Here's how the part is built. I have some questions about the finished solid (model axes, mm). A direction names the side the tool comes from. Coordinates: 2 decimals unless noted, no trailing zeros. Order: outer loops, then holes, each group sorted by start corner. A loop starts at its lowest first (then second) coordinate and runs counter-clockwise, first axis right, second up. Notation, with made-up numbers: (-17.75, 8) - (28.25, 8) arc R9 ccw to (28.25, 12) - close; hole circle Ø1 at (48, 76.5). An arc over 180 degrees is marked (long way). Answer as CSV lines item,"result". Start each with the question number.
Q1. Suppose I cut it at B-B (x = 3.5). Please give me the cut outline in (y, z).
Q2. For faces 1 (the face through (-4, 4, 35)), 2 (the face through (-5, 0, 44.85)), 3 (the face through (3, 0, 59.85)), which set-ups out of +Z, -Z, +X, -X, +Y, -Y let a thin tool reach every point of the face, with its end or its side?
Q3. Suppose I cut it at A-A (y = -3.75). Please give me the cut outline in (x, z), then the cut area to 3 significant figures.
Q4. Suppose I cut it at C-C (z = 20). Please give me the cut outline in (x, y).
Q5. Suppose I cut it at D-D (z = 54.5). Please give me the cut outline in (x, y).
Q6. Thinking about a two-plate mould opening in Y: for faces 4 (the face through (-1.08, 4.88, 17.26)), 5 (the face through (2.44, 0.54, 55.79)), 6 (the face through (-4, 0, 52)), 7 (the face through (-0.424, 0.094, 50.609)), which applies, released by +Y, released by -Y, zero draft, split by the parting line, or undercut?
Q7. I need wall thicknesses on line 1 (X direction, y = 0, z = 56.25); line 2 (Y direction, x = 0, z = 54.25); line 3 (Z direction, x = -4.75, y = 3.25). Which ranges of each line are inside material? Lowest first, please.
Q8. For pin 1 Ø3.5 at (x, y) = (1, 1.5) entering from -Z; pin 2 Ø7 at (y, z) = (0.5, 51) entering from -X; pin 3 Ø4 at (y, z) = (-4, 27) entering from -X, each with a flat end and sliding along its axis, tell me the tip position at first contact or that it passes through.
Autodesk Inventor part; units mm, degrees
ref_plane "作業平面1" through (0, 6, 59.85) normal (0, 1, 0) x (-1, 0, 0)
ref_plane "YZ Plane" through (0, 0, 0) normal (1, 0, 0) x (0, 1, 0)
ref_plane "XZ Plane" through (0, 0, 0) normal (0, 1, 0) x (-1, 0, 0)
sketch "スケッチ1" plane through (0, 0, 0) normal (0, 0, 1) x (1, 0, 0)
  point P0 (0, 0)
sketch "スケッチ2" plane through (0, 0, 0) normal (0, 0, 1) x (1, 0, 0)
  circle A0 centre (0, 0) radius 5
  dimension "d0" = 10
extrude "押し出し1" add sketch "スケッチ2" along normal blind 35
thread "ねじ1"
sketch "スケッチ3" plane through (0, 0, 35) normal (0, 0, 1) x (1, 0, 0)
  point P0 (0, 0)
sketch "スケッチ4" plane through (0, 0, 35) normal (0, 0, 1) x (1, 0, 0)
  circle A0 centre (0, 0) radius 6
  dimension "d5" = 12
extrude "押し出し2" add sketch "スケッチ4" along normal blind 24.85
sketch "スケッチ5" plane through (0, 0, 59.85) normal (0, 0, 1) x (1, 0, 0)
  line L0 (0, 0) -> (0, 6)
  circle A0 centre (0, 0) radius 6
ref_plane "作業平面1" through (0, 6, 59.85) normal (0, 1, 0) x (-1, 0, 0)
sketch "スケッチ9" plane through (0, 0, 59.85) normal (0, 0, 1) x (1, 0, 0)
  point P0 (0, 0)
  point P1 (0, 0)
hole "穴2" at (0, 0, 59.85) direction (0, 0, -1) diameter 5 depth 8 tip angle 118
thread "ねじ3"
sketch "スケッチ10" plane through (0, 0, 59.85) normal (0, 0, 1) x (1, 0, 0)
  arc A0 (-4, 4.4721) -> (-4, -4.4721) centre (0, 0) ccw
  line L0 (-4, 0) -> (-4, 4.4721)
  line L1 (-4, 0) -> (-4, -4.4721)
  dimension "d34" = 12
  dimension "d35" = 4
extrude "押し出し4" cut sketch "スケッチ10" against normal blind 15
properties part number "回転アーム付き計測輪シャフト"
Here are the results:
1,outline,"(-4.87, 35) - (-3.57, 35) - (-3.57, 0) - (3.57, 0) - (3.57, 35) - (4.87, 35) - (4.87, 59.85) - (-4.87, 59.85) - close"
2,face 1,"-Z"
2,face 2,"+Z, -X, +Y, -Y"
2,face 3,"+Z, +X, -X, +Y, -Y"
3,outline,"(-4.68, 35) - (-3.31, 35) - (-3.31, 0) - (3.31, 0) - (3.31, 35) - (4.68, 35) - (4.68, 59.85) - (-4, 59.85) - (-4, 44.85) - (-4.68, 44.85) - close"
3,area,"454 mm²"
4,outline,"circle Ø10 at (0, 0)"
5,outline,"(-4, -4.47) arc R6 ccw (long way) to (-4, 4.47) - close; hole circle Ø5 at (0, 0)"
6,face 4,"split by the parting line"
6,face 5,"undercut"
6,face 6,"zero draft"
6,face 7,"undercut"
7,line 1,"x = -4 to -2.5, 2.5 to 6"
7,line 2,"y = -6 to -2.5, 2.5 to 6"
7,line 3,"z = 35 to 44.85"
8,pin 1,"stops at z = 0"
8,pin 2,"stops at x = -4"
8,pin 3,"stops at x = -4.58"
